For this review, use the dimensioned drawing (mm, ordinates from the lowest corner) and the shaded views. A direction names the side the tool comes from. Round coordinates to 2 decimals unless told otherwise and drop trailing zeros. Loops run counter-clockwise (first coordinate to the right, second up) from the corner with the lowest first, then second, coordinate; pieces in that order, holes last. Notation, with made-up numbers: (-14, -37.75) - (-2, -37.75) arc R16 ccw to (-2, -12.75) - close; hole circle Ø3 at (20, 0). An arc over 180 degrees is marked (long way). Answer as CSV lines item,"result". Start each with the question number.
(1) Wall thickness on L1, parallel to Y at x = 30, z = 3.3; L2, parallel to X at y = 24.5, z = 1.4; L3, parallel to Y at x = 55, z = 2.65: over which ranges is each line inside the solid? List them lowest first.
(2) For P1, Ø1, axis at x = 42.5, y = 19, coming from the -Z side; P2, Ø4, axis at x = 5, y = 26, coming from the -Z side; P3, Ø2, axis at x = 28, z = 2, coming from the +Y side, all flat-tipped, find the tip position at first contact; note any pin that passes through.
(3) Consider section B-B (x = 40). Give the boundary of the cut face in (y, z), and give its area (3 significant figures).
(4) For the marked faces 1 and 2, list the 3-axis set-ups (+Z, -Z, +X, -X, +Y, -Y) from which the entire face can be reached by the end or side of a thin tool; tool diameter is ignored.
(5) Consider section A-A (z = 0.7). Give the boundary of the cut face in (x, y), and give its area (3 significant figures).
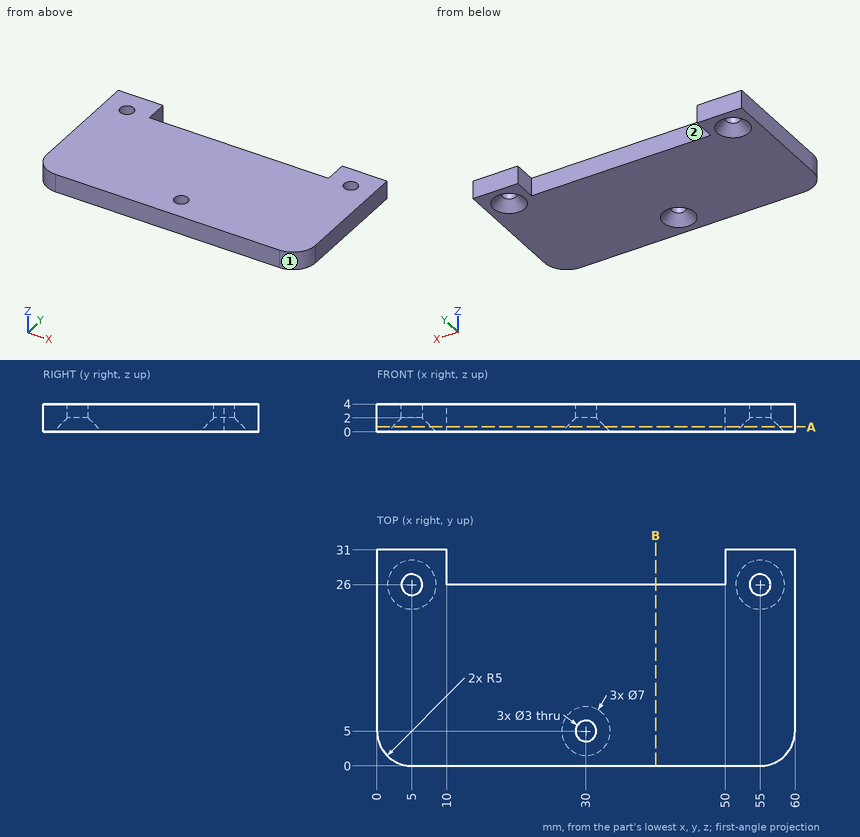
Determined:
1,L1,"y = 0 to 3.5, 6.5 to 26"
1,L2,"x = 0 to 3.53, 6.47 to 53.53, 56.47 to 60"
1,L3,"y = 0 to 24.5, 27.5 to 31"
2,P1,"stops at z = 0"
2,P2,"stops at z = 1.5"
2,P3,"stops at y = 26"
3,outline,"(0, 0) - (26, 0) - (26, 4) - (0, 4) - close"
3,area,"104 mm^2"
4,face 1,"+Z, -Z, +X, -Y"
4,face 2,"+Z, -Z, +Y"
5,outline,"(0, 5) arc R5 ccw to (5, 0) - (55, 0) arc R5 ccw to (60, 5) - (60, 31) - (50, 31) - (50, 26) - (10, 26) - (10, 31) - (0, 31) - close; hole circle Ø5.6 at (5, 26); hole circle Ø5.6 at (30, 5); hole circle Ø5.6 at (55, 26)"
5,area,"1,580 mm^2"
